Job drawing, mm, ordinate dimensions from the low corner. One solid piece. A direction names the side the tool comes from. Coordinates: 2 decimals unless noted, no trailing zeros. Write each loop counter-clockwise with the first axis right and the second up, starting at its lowest first coordinate (ties: lowest second). Pieces come first, ordered by that corner, then holes.
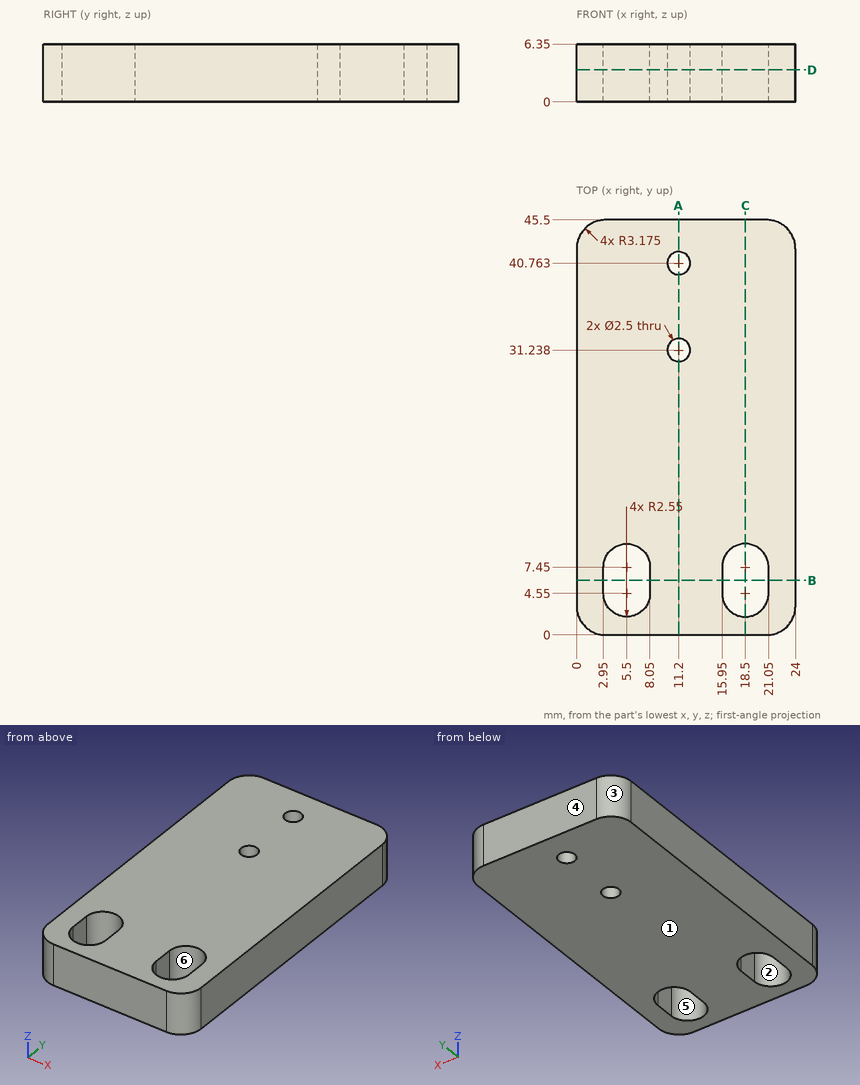
1. Flat gauge pin, fed straight in: pin 1 (2 mm diameter, centred on x = 11.2, y = 31.24, fed in from -Z). Where does the tip first touch, or does it go through?
Computed values:
pin 1: passes through
2. 3-axis set-ups, long thin cutter, end or side, ignore diameter. For the marked faces 1 and 2: which of +Z, -Z, +X, -X, +Y, -Y reach the whole face in a straight line?
Computed values:
face 1: -Z, +X, -X, +Y, -Y
face 2: +Z, -Z
3. Saw through at C-C on x = 18.5. List the corners of the cut face in (y, z).
Computed values:
outline: (0, 0) - (2, 0) - (2, 6.35) - (0, 6.35) - close; (10, 0) - (45.5, 0) - (45.5, 6.35) - (10, 6.35) - close
4. Probe line 1 along X through (y, z) = (7, 5.5); line 2 along Y through (x, z) = (11.2, 2.5); line 3 along X through (y, z) = (9.5, 3.5) (1 decimal). List the from-to ranges inside material, lowest first.
Computed values:
line 1: x = 0 to 2.95, 8.05 to 15.95, 21.05 to 24
line 2: y = 0 to 29.99, 32.49 to 39.51, 42.01 to 45.5
line 3: x = 0 to 4, 7 to 17, 20 to 24
5. Saw through at D-D on z = 3.5. State how many separate pieces and enclosed holes the cut face has, plus the area to 3 significant figures.
Computed values:
separate pieces: 1
enclosed holes: 4
area: 1,000 mm2
6. Saw through at A-A on x = 11.2. List the corners of the cut face in (y, z).
Computed values:
outline: (0, 0) - (29.99, 0) - (29.99, 6.35) - (0, 6.35) - close; (32.49, 0) - (39.51, 0) - (39.51, 6.35) - (32.49, 6.35) - close; (42.01, 0) - (45.5, 0) - (45.5, 6.35) - (42.01, 6.35) - close
7. Saw through at B-B on y = 6. List the corners of the cut face in (x, z).
Computed values:
outline: (0, 0) - (2.95, 0) - (2.95, 6.35) - (0, 6.35) - close; (8.05, 0) - (15.95, 0) - (15.95, 6.35) - (8.05, 6.35) - close; (21.05, 0) - (24, 0) - (24, 6.35) - (21.05, 6.35) - close
8. Mould opens along X. For the marked faces 3, 4, 5 and 6 say: +X half, -X half, draft (parallel to the pull), parting line (faces both ways), or undercut.
Computed values:
face 3: -X half
face 4: draft
face 5: undercut
face 6: undercut
